Autodesk Inventor part; units mm, degrees
ref_plane "YZ Plane" through (0, 0, 0) normal (1, 0, 0) x (0, 1, 0)
ref_plane "XZ Plane" through (0, 0, 0) normal (0, 1, 0) x (-1, 0, 0)
ref_plane "XY Plane" through (0, 0, 0) normal (0, 0, 1) x (1, 0, 0)
sketch "Sketch1" plane through (0, 0, 0) normal (0, 1, 0) x (-1, 0, 0)
  line L0 (9.8, 0) -> (-9.8, 0)
  line L1 (0, -35) -> (0, 35)
  line L2 (7, 25) -> (-7, 25)
  line L3 (-7, -25) -> (7, -25)
  line L4 (7, -25) -> (7, 25)
  line L5 (-7, 12) -> (-1, 12)
  line L6 (-1, 12) -> (-1, 6)
  line L7 (-1, 6) -> (-7, 6)
  line L8 (-7, 25) -> (-7, 12)
  line L9 (-7, 6) -> (-7, -25)
  point P0 (0, 0)
  point P1 (7, 0)
  point P2 (0, 25)
  dimension "d0" = 14
  dimension "d1" = 50
  dimension "d2" = 6
  dimension "d3" = 6
  dimension "d4" = 13
extrude "Extrusion1" add sketch "Sketch1" along normal blind 30
properties part number "FP Rear Hood"
Geometry: final body of the model. Coordinates: model frame, mm. A direction names the side the tool comes from. Round coordinates to 2 decimals unless told otherwise and drop trailing zeros. Loops run counter-clockwise (first coordinate to the right, second up) from the corner with the lowest first, then second, coordinate; pieces in that order, holes last.
Item 1: Section A-A, the plane x = 4.75. Output: boundary loops of the cut face in (y, z), plus the area to 3 significant figures.
Checked values:
outline: (0, -25) - (30, -25) - (30, 6) - (0, 6) - close; (0, 12) - (30, 12) - (30, 25) - (0, 25) - close
area: 1,320 mm2
Item 2: Mould query, pull axis Z, two halves, no side actions, for faces 3 (the flat face through (4, 15, 12)), 4 (the flat face through (0, 30, 0)), 5 (the flat face through (0, 15, -25)), 6 (the flat face through (1, 15, 9)). Classes: released by +Z, released by -Z, zero draft, split by the parting line, or undercut.
Checked values:
face 3: undercut
face 4: zero draft
face 5: released by -Z
face 6: undercut
Item 3: Contact query for a flat-ended pin moving along its axis: P1, Ø3, axis at y = 9.5, z = 9.5, coming from the +X side. Output: stop coordinate, or through.
Checked values:
P1: stops at x = 1
Item 4: Section B-B, the plane y = 14.5. Output: boundary loops of the cut face in (x, z), plus the area to 3 significant figures.
Checked values:
outline: (-7, -25) - (7, -25) - (7, 6) - (1, 6) - (1, 12) - (7, 12) - (7, 25) - (-7, 25) - close
area: 664 mm2
Item 5: Line query: L1, parallel to Z at x = 2, y = 4.75; L2, parallel to X at y = 7.5, z = 10.5. Output: solid intervals per line, ascending.
Checked values:
L1: z = -25 to 6, 12 to 25
L2: x = -7 to 1
Item 6: Reachability of faces 1 (the flat face through (4, 15, 6)), 2 (the flat face through (-7, 15, 0)) from +Z, -Z, +X, -X, +Y, -Y: full face, straight path, thin tool, end or side. Return the list, or none.
Checked values:
face 1: +X, +Y, -Y
face 2: +Z, -Z, -X, +Y, -Y
